Input: part model. Units: mm. Frame: model coordinates. A direction names the side the tool comes from. Coordinates: 2 decimals unless noted, no trailing zeros.
Item 1: Reachability of faces 1 (the flat face through (9, -254, 17)), 2 (the flat face through (9, -254, 1)), 3 (the flat face through (139, 0, 9)) from +Z, -Z, +X, -X, +Y, -Y: full face, straight path, thin tool, end or side. Return the list, or none.
Item 2: Contact query for flat-ended pins moving along their axis: P1, Ø3, axis at y = -194.5, z = 7.5, coming from the -X side; P2, Ø2, axis at x = 20, z = 9, coming from the +Y side; P3, Ø0.5, axis at y = -240.5, z = 0.5, coming from the -X side; P4, Ø2, axis at x = 141, z = 9, coming from the -Y side. Output: stop coordinate, or through.
Item 3: Ray query, line 1 along X through (y, z) = (-9.75, 9); line 2 along Z through (x, y) = (20, -3.5); line 3 along X through (y, z) = (-21.5, 0.5). Return the intervals inside material, ascending.
```python
from build123d import *

# Parameters (mm, degrees)
F0_W     = 282
F0_H     = 500
F1_DEPTH = 18
F3_D     = 2.5
F3_DEPTH = 14.5
F3_TIP   = 0.7510757738
F5_D     = 2.5
F5_DEPTH = 14
F5_TIP   = 0.7510757738
F6_W     = 18
F6_H     = 1
F7_DEPTH = 500.001


with BuildPart() as f1:
    # F0 (on Top) → F1 (new body)
    with BuildSketch(Plane.XY):
        with Locations((141, -250)):
            Rectangle(F0_W, F0_H)
    extrude(amount=F1_DEPTH)

    # F3
    with Locations(Plane.XZ.offset(500)):
        with Locations((20, 9), (141, 9), (262, 9)):
            Hole(F3_D / 2, depth=F3_DEPTH)
            with Locations((0, 0, -(F3_DEPTH + F3_TIP / 2))):  # 118° drill point
                Cone(0, F3_D / 2, F3_TIP, mode=Mode.SUBTRACT)

    # F5
    with Locations(Plane(origin=(0, 0, 0), x_dir=(-1, 0, 0), z_dir=(0, 1, 0))):
        with Locations((-262, 9), (-141, 9), (-20, 9)):
            Hole(F5_D / 2, depth=F5_DEPTH)
            with Locations((0, 0, -(F5_DEPTH + F5_TIP / 2))):  # 118° drill point
                Cone(0, F5_D / 2, F5_TIP, mode=Mode.SUBTRACT)

    # F6 (on face) → F7 (cut, through all)
    with BuildSketch(Plane.XZ.offset(500)):
        with Locations((9, 17.5)):
            Rectangle(F6_W, F6_H)
        with Locations((9, 0.5)):
            Rectangle(F6_W, F6_H)
    extrude(amount=-F7_DEPTH, mode=Mode.SUBTRACT)


solid = f1.part
```
Results found:
1. face 1: +Z, -X, +Y, -Y
1. face 2: -Z, -X, +Y, -Y
1. face 3: +Z, -Z, +X, -X, +Y
2. P1: stops at x = 0
2. P2: stops at y = -14.15
2. P3: stops at x = 18
2. P4: stops at y = -485.35
3. line 1: x = 0 to 18.75, 21.25 to 139.75, 142.25 to 260.75, 263.25 to 282
3. line 2: z = 0 to 7.75, 10.25 to 18
3. line 3: x = 18 to 282
